```python
from build123d import *

# Parameters (mm, degrees)
EXTRUDE_1_DEPTH     = 3
SKETCH_3_R          = 3.25
CUT_EXTRUDE_1_DEPTH = 1
EXTRUDE_START       = -0.5
EXTRUDE_2_DEPTH     = 10
SKETCH_5_OUTSIDE_W  = 43.322
SKETCH_5_OUTSIDE_H  = 35.322
CUT_EXTRUDE_2_DEPTH = 22.122026418
FILLET_1_R          = 1
SKETCH_6_R          = 1.6
CUT_EXTRUDE_3_DEPTH = 20.972230797


# Read off the part's stored shape, not the designer's step: 凸台-拉伸1
with BuildPart() as part:
    # 凸台-拉伸1 outline → 凸台-拉伸1 (new body)
    with BuildSketch(Plane.XY):
        with BuildLine():
            Line((15, -5.5), (15, 5.5))
            Line((15, 5.5), (1.899494937, 5.5))
            Line((1.899494937, 5.5), (-4.075378798, 11.474873734))
            ThreePointArc((-4.075378798, 11.474873734), (-6.550252532, 12.5), (-9.025126266, 11.474873734))
            Line((-9.025126266, 11.474873734), (-15, 5.5))
            Line((-15, 5.5), (-15, -5.5))
            Line((-15, -5.5), (-1.899494937, -5.5))
            Line((-1.899494937, -5.5), (4.075378798, -11.474873734))
            ThreePointArc((4.075378798, -11.474873734), (6.550252532, -12.5), (9.025126266, -11.474873734))
            Line((9.025126266, -11.474873734), (15, -5.5))
        make_face()
    extrude(amount=EXTRUDE_1_DEPTH)

    # 草图3 → 切除-拉伸1 (cut)
    with BuildSketch(Plane.XY.offset(3)):
        with Locations((-6.550252532, 9)):
            Circle(SKETCH_3_R)
        with Locations((6.550252532, -9)):
            Circle(SKETCH_3_R)
    extrude(amount=-CUT_EXTRUDE_1_DEPTH, mode=Mode.SUBTRACT)

    # 草图4 → 凸台-拉伸2 (add)
    with BuildSketch(Plane(origin=(0, 5.5, 0), x_dir=(1, 0, 0), z_dir=(0, 1, 0)).offset(EXTRUDE_START)):
        with BuildLine():
            Line((-16.16, 1.2), (-16.5, 1.2))
            Line((-16.5, 1.2), (-16.5, -0.977568186))
            Line((-16.5, -0.977568186), (16.5, -0.977568186))
            Line((16.5, -0.977568186), (16.5, 1.2))
            Line((16.5, 1.2), (16.16, 1.2))
            ThreePointArc((16.16, 1.2), (15.976152237, 1.123847763), (15.9, 0.94))
            Line((15.9, 0.94), (15.9, 0.9))
            ThreePointArc((15.9, 0.9), (15, 0), (14.1, 0.9))
            Line((14.1, 0.9), (14.1, 0.94))
            ThreePointArc((14.1, 0.94), (14.023847763, 1.123847763), (13.84, 1.2))
            Line((13.84, 1.2), (13.5, 1.2))
            Line((13.5, 1.2), (13.16, 1.2))
            ThreePointArc((13.16, 1.2), (12.976152237, 1.123847763), (12.9, 0.94))
            Line((12.9, 0.94), (12.9, 0.9))
            ThreePointArc((12.9, 0.9), (12, 0), (11.1, 0.9))
            Line((11.1, 0.9), (11.1, 0.94))
            ThreePointArc((11.1, 0.94), (11.023847763, 1.123847763), (10.84, 1.2))
            Line((10.84, 1.2), (10.5, 1.2))
            Line((10.5, 1.2), (10.16, 1.2))
            ThreePointArc((10.16, 1.2), (9.976152237, 1.123847763), (9.9, 0.94))
            Line((9.9, 0.94), (9.9, 0.9))
            ThreePointArc((9.9, 0.9), (9, 0), (8.1, 0.9))
            Line((8.1, 0.9), (8.1, 0.94))
            ThreePointArc((8.1, 0.94), (8.023847763, 1.123847763), (7.84, 1.2))
            Line((7.84, 1.2), (7.5, 1.2))
            Line((7.5, 1.2), (7.16, 1.2))
            ThreePointArc((7.16, 1.2), (6.976152237, 1.123847763), (6.9, 0.94))
            Line((6.9, 0.94), (6.9, 0.9))
            ThreePointArc((6.9, 0.9), (6, 0), (5.1, 0.9))
            Line((5.1, 0.9), (5.1, 0.94))
            ThreePointArc((5.1, 0.94), (5.023847763, 1.123847763), (4.84, 1.2))
            Line((4.84, 1.2), (4.5, 1.2))
            Line((4.5, 1.2), (4.16, 1.2))
            ThreePointArc((4.16, 1.2), (3.976152237, 1.123847763), (3.9, 0.94))
            Line((3.9, 0.94), (3.9, 0.9))
            ThreePointArc((3.9, 0.9), (3, 0), (2.1, 0.9))
            Line((2.1, 0.9), (2.1, 0.94))
            ThreePointArc((2.1, 0.94), (2.023847763, 1.123847763), (1.84, 1.2))
            Line((1.84, 1.2), (1.5, 1.2))
            Line((1.5, 1.2), (1.16, 1.2))
            ThreePointArc((1.16, 1.2), (0.976152237, 1.123847763), (0.9, 0.94))
            Line((0.9, 0.94), (0.9, 0.9))
            ThreePointArc((0.9, 0.9), (0, 0), (-0.9, 0.9))
            Line((-0.9, 0.9), (-0.9, 0.94))
            ThreePointArc((-0.9, 0.94), (-0.976152237, 1.123847763), (-1.16, 1.2))
            Line((-1.16, 1.2), (-1.5, 1.2))
            Line((-1.5, 1.2), (-1.84, 1.2))
            ThreePointArc((-1.84, 1.2), (-2.023847763, 1.123847763), (-2.1, 0.94))
            Line((-2.1, 0.94), (-2.1, 0.9))
            ThreePointArc((-2.1, 0.9), (-3, 0), (-3.9, 0.9))
            Line((-3.9, 0.9), (-3.9, 0.94))
            ThreePointArc((-3.9, 0.94), (-3.976152237, 1.123847763), (-4.16, 1.2))
            Line((-4.16, 1.2), (-4.5, 1.2))
            Line((-4.5, 1.2), (-4.84, 1.2))
            ThreePointArc((-4.84, 1.2), (-5.023847763, 1.123847763), (-5.1, 0.94))
            Line((-5.1, 0.94), (-5.1, 0.9))
            ThreePointArc((-5.1, 0.9), (-6, 0), (-6.9, 0.9))
            Line((-6.9, 0.9), (-6.9, 0.94))
            ThreePointArc((-6.9, 0.94), (-6.976152237, 1.123847763), (-7.16, 1.2))
            Line((-7.16, 1.2), (-7.5, 1.2))
            Line((-7.5, 1.2), (-7.84, 1.2))
            ThreePointArc((-7.84, 1.2), (-8.023847763, 1.123847763), (-8.1, 0.94))
            Line((-8.1, 0.94), (-8.1, 0.9))
            ThreePointArc((-8.1, 0.9), (-9, 0), (-9.9, 0.9))
            Line((-9.9, 0.9), (-9.9, 0.94))
            ThreePointArc((-9.9, 0.94), (-9.976152237, 1.123847763), (-10.16, 1.2))
            Line((-10.16, 1.2), (-10.5, 1.2))
            Line((-10.5, 1.2), (-10.84, 1.2))
            ThreePointArc((-10.84, 1.2), (-11.023847763, 1.123847763), (-11.1, 0.94))
            Line((-11.1, 0.94), (-11.1, 0.9))
            ThreePointArc((-11.1, 0.9), (-12, 0), (-12.9, 0.9))
            Line((-12.9, 0.9), (-12.9, 0.94))
            ThreePointArc((-12.9, 0.94), (-12.976152237, 1.123847763), (-13.16, 1.2))
            Line((-13.16, 1.2), (-13.5, 1.2))
            Line((-13.5, 1.2), (-13.84, 1.2))
            ThreePointArc((-13.84, 1.2), (-14.023847763, 1.123847763), (-14.1, 0.94))
            Line((-14.1, 0.94), (-14.1, 0.9))
            ThreePointArc((-14.1, 0.9), (-15, 0), (-15.9, 0.9))
            Line((-15.9, 0.9), (-15.9, 0.94))
            ThreePointArc((-15.9, 0.94), (-15.976152237, 1.123847763), (-16.16, 1.2))
        make_face()
    extrude(amount=-EXTRUDE_2_DEPTH)

    # 草图5 outside → 切除-拉伸2 (cut, through all)
    with BuildSketch(Plane.XY.offset(3)):
        Rectangle(SKETCH_5_OUTSIDE_W, SKETCH_5_OUTSIDE_H)
        with BuildLine():
            Line((15, -5.5), (15, 5.5))
            Line((15, 5.5), (1.899494937, 5.5))
            Line((1.899494937, 5.5), (-4.075378798, 11.474873734))
            ThreePointArc((-4.075378798, 11.474873734), (-6.550252532, 12.5), (-9.025126266, 11.474873734))
            Line((-9.025126266, 11.474873734), (-15, 5.5))
            Line((-15, 5.5), (-15, -5.5))
            Line((-15, -5.5), (-1.899494937, -5.5))
            Line((-1.899494937, -5.5), (4.075378798, -11.474873734))
            ThreePointArc((4.075378798, -11.474873734), (6.550252532, -12.5), (9.025126266, -11.474873734))
            Line((9.025126266, -11.474873734), (15, -5.5))
        make_face(mode=Mode.SUBTRACT)
    extrude(amount=-CUT_EXTRUDE_2_DEPTH, mode=Mode.SUBTRACT)

    # 圆角1
    # the kernel refuses this fillet: 1 mm, written as the material it takes off along each edge
    with BuildSketch(Plane(origin=(15, -5.5, -1.035533906), x_dir=(-0.7071067811865454, -0.7071067811865497, 0), z_dir=(0, 0, 1))) as fillet_1_piece_1:
        with BuildLine():
            CenterArc((FILLET_1_R * 0.414213562373, -FILLET_1_R), FILLET_1_R, 90, 45)
            Line((-FILLET_1_R * 0.292893218813, -FILLET_1_R * 0.292893218813), (0, 0))
            Line((0, 0), (FILLET_1_R * 0.414213562373, 0))
        make_face()
    extrude(amount=5.071067812, mode=Mode.SUBTRACT)
    with BuildSketch(Plane(origin=(-15, -5.5, -2.5), x_dir=(1, 0, 0), z_dir=(0, 0, 1))) as fillet_1_piece_2:
        with BuildLine():
            CenterArc((FILLET_1_R, FILLET_1_R), FILLET_1_R, 180, 90)
            Line((0, FILLET_1_R), (0, 0))
            Line((0, 0), (FILLET_1_R, 0))
        make_face()
    extrude(amount=8, mode=Mode.SUBTRACT)
    with BuildSketch(Plane(origin=(-15, 5.5, -1.035533906), x_dir=(0, -1, 0), z_dir=(0, 0, 1))) as fillet_1_piece_3:
        with BuildLine():
            CenterArc((FILLET_1_R * 0.414213562373, FILLET_1_R), FILLET_1_R, 225, 45)
            Line((-FILLET_1_R * 0.292893218813, FILLET_1_R * 0.292893218813), (0, 0))
            Line((0, 0), (FILLET_1_R * 0.414213562373, 0))
        make_face()
    extrude(amount=5.071067812, mode=Mode.SUBTRACT)
    with BuildSketch(Plane(origin=(15, 5.5, -2.5), x_dir=(0, -1, 0), z_dir=(0, 0, 1))) as fillet_1_piece_4:
        with BuildLine():
            CenterArc((FILLET_1_R, -FILLET_1_R), FILLET_1_R, 90, 90)
            Line((0, -FILLET_1_R), (0, 0))
            Line((0, 0), (FILLET_1_R, 0))
        make_face()
    extrude(amount=8, mode=Mode.SUBTRACT)

    # 草图6 → 切除-拉伸3 (cut, through all)
    with BuildSketch(Plane.XY.offset(3)):
        with Locations((-6.550252532, 9)):
            Circle(SKETCH_6_R)
        with Locations((6.550252532, -9)):
            Circle(SKETCH_6_R)
    extrude(amount=-CUT_EXTRUDE_3_DEPTH, mode=Mode.SUBTRACT)


solid = part.part
```
Part model, mm, in its own coordinate system. A direction names the side the tool comes from. Round coordinates to 2 decimals unless told otherwise and drop trailing zeros. Write each loop counter-clockwise with the first axis right and the second up, starting at its lowest first coordinate (ties: lowest second). Pieces come first, ordered by that corner, then holes. Notation, with made-up numbers: M 13.25,31 L 68.25,31 A26 cw 68.25,66 Z; hole C -25.5,24.5 d11. An arc over 180 degrees is marked long. Answer as CSV lines item,"result". Start each with the question number.
1) Drill centre lines: L1, parallel to Y at x = -5, z = -0.3; L2, parallel to Z at x = -11, y = 6.25; L3, parallel to Z at x = 6, y = -7.25. Where is each one in solid material? Low to high.
2) Drop flat-ended pins along their axis: pin 1 (1.5 mm diameter, centred on x = -9, z = 0, fed in from +Y); pin 2 (0.6 mm diameter, centred on x = -7, z = -0.5, fed in from -Y); pin 3 (0.6 mm diameter, centred on x = -14, z = -1, fed in from +Y). Give the stop position or say it passes through.
3) Mould opens along Y. For faces 1 (the face through (-1.5, 5, -0.5)), 2 (the face through (-6.9, 7.44, 1.01)), 3 (the face through (6.5, -12.5, 1.5)) say: +Y half, -Y half, draft (parallel to the pull), parting line (faces both ways), or undercut.
4) Band-saw the part on B-B (y = 8). List the corners of the cut face in (x, z).
5) Band-saw the part on D-D (y = -7). List the corners of the cut face in (x, z).
6) Band-saw the part on C-C (x = -10.5). List the corners of the cut face in (y, z).
7) Which spindle directions (+Z, -Z, +X, -X, +Y, -Y) get a long thin tool onto all of the face, cutting with end or side? Do faces 4 (the face through (-13.5, 5, -0.5)), 5 (the face through (-15, 0, 1)), 6 (the face through (10.5, -5, -0.5)). Say none if no direction does.
8) Band-saw the part on A-A (z = 1.6). List the corners of the cut face in (x, y).
Worked out:
1,L1,"-5 to 5"
1,L2,"0 to 3"
1,L3,"0 to 2"
2,pin 1,"y = 12.06"
2,pin 2,"y = -5"
2,pin 3,"y = 5"
3,face 1,"+Y half"
3,face 2,"undercut"
3,face 3,"-Y half"
4,outline,"M -12.5,0 L -7.8,0 L -7.8,2 L -9.64,2 L -9.64,3 L -12.5,3 Z; M -5.3,0 L -0.6,0 L -0.6,3 L -3.46,3 L -3.46,2 L -5.3,2 Z"
5,outline,"M -0.4,0 L 13.5,0 L 13.5,3 L 9.11,3 L 9.11,2 L 3.99,2 L 3.99,3 L -0.4,3 Z"
6,outline,"M -5.5,0 L -5,0 L -5,-1.2 L 5,-1.2 L 5,0 L 10,0 L 10,3 L -5.5,3 Z"
7,face 4,"-Z, +X, -X, +Y"
7,face 5,"+Z, -Z, -X, +Y, -Y"
7,face 6,"-Z, +X, -X, -Y"
8,outline,"M -15,-4.5 A1 ccw -14,-5.5 L -1.9,-5.5 L 4.08,-11.47 A3.5 ccw 9.03,-11.47 L 14.71,-5.79 A1 ccw 15,-5.09 L 15,4.5 A1 ccw 14,5.5 L 1.9,5.5 L -4.08,11.47 A3.5 ccw -9.03,11.47 L -14.71,5.79 A1 ccw -15,5.09 Z; hole C -6.55,9 d3.2; hole C 6.55,-9 d3.2"
